Part print with two shaded views. Sizes in mm from the minimum x, y, z corner. A direction names the side the tool comes from. Give positions to 0.01 mm unless a question says otherwise; leave off trailing zeros. Write each loop counter-clockwise with the first axis right and the second up, starting at its lowest first coordinate (ties: lowest second). Pieces come first, ordered by that corner, then holes.
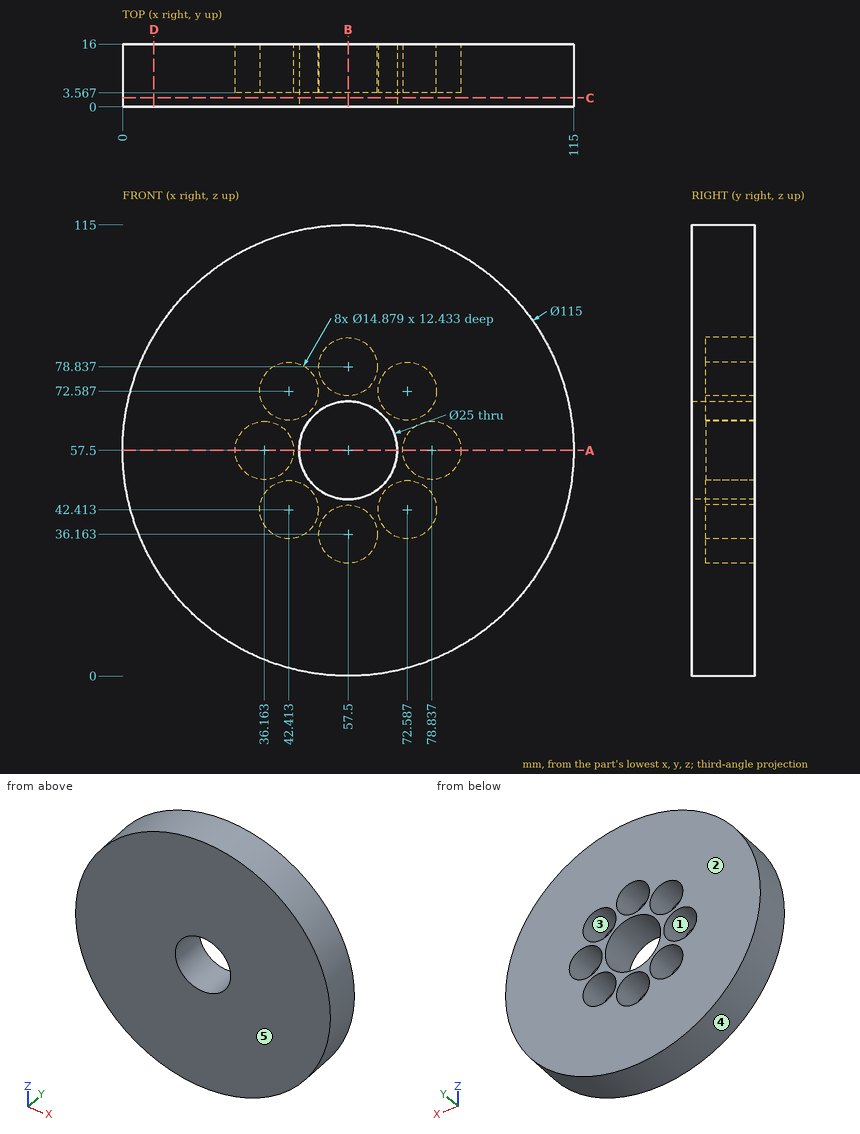
1) 3-axis set-ups, long thin cutter, end or side, ignore diameter. For the marked faces 1 and 2: which of +Z, -Z, +X, -X, +Y, -Y reach the whole face in a straight line?
Answers follow:
face 1: +Y
face 2: +Z, -Z, +X, -X, +Y
2) Saw through at A-A, the plane z = 57.5. Write the cut outline in (x, y) (1 decimal), then the cut area to 3 significant figures.
Answers follow:
outline: (0, 0) - (45, 0) - (45, 16) - (43.6, 16) - (43.6, 3.6) - (28.7, 3.6) - (28.7, 16) - (0, 16) - close; (70, 0) - (115, 0) - (115, 16) - (86.3, 16) - (86.3, 3.6) - (71.4, 3.6) - (71.4, 16) - (70, 16) - close
area: 1,070 mm2
3) Two-plate mould, pull along Z, no slides. Class the marked faces 3, 4 and 5: +Z half, -Z half, draft (parallel to the pull), parting line (faces both ways), or undercut.
Answers follow:
face 3: undercut
face 4: parting line
face 5: draft
4) Saw through at C-C, the plane y = 2.25. Write the cut outline in (x, z), then the cut area to 3 significant figures.
Answers follow:
outline: circle Ø115 at (57.5, 57.5); hole circle Ø25 at (57.5, 57.5)
area: 9,900 mm2
5) Pin check, flat tips, straight feed: pin 1 Ø17 at (x, z) = (72.59, 42.41) entering from -Y; pin 2 Ø3 at (y, z) = (14, 44) entering from -X; pin 3 Ø7.5 at (x, z) = (40.5, 75.5) entering from +Y; pin 4 Ø1 at (x, y) = (81, 6) entering from -Z. Stop position of each tip, or through.
Answers follow:
pin 1: stops at y = 0
pin 2: stops at x = 1.27
pin 3: stops at y = 3.57
pin 4: stops at z = 4.8
6) Saw through at D-D, the plane x = 8. Write the cut outline in (y, z).
Answers follow:
outline: (0, 28.24) - (16, 28.24) - (16, 86.76) - (0, 86.76) - close
7) Wall check: L1, parallel to X at y = 9, z = 57.5 (1 decimal); L2, parallel to Z at x = 73, y = 6 (1 decimal); L3, parallel to Z at x = 67.5, y = 4.25 (1 decimal). Give the ranges that are in metal, low to high.
Answers follow:
L1: x = 0 to 28.7, 43.6 to 45, 70 to 71.4, 86.3 to 115
L2: z = 2.1 to 35, 49.8 to 52.9, 62.1 to 65.2, 80 to 112.9
L3: z = 0.9 to 37, 47.8 to 50, 65 to 67.2, 78 to 114.1
8) Saw through at B-B, the plane x = 57.5. Write the cut outline in (y, z) (1 decimal), then the cut area to 3 significant figures.
Answers follow:
outline: (0, 0) - (16, 0) - (16, 28.7) - (3.6, 28.7) - (3.6, 43.6) - (16, 43.6) - (16, 45) - (0, 45) - close; (0, 70) - (16, 70) - (16, 71.4) - (3.6, 71.4) - (3.6, 86.3) - (16, 86.3) - (16, 115) - (0, 115) - close
area: 1,070 mm2
